The drawing under review shows one solid part. Ordinate dimensions are in mm from its lowest x, y, z. A direction names the side the tool comes from. Give positions to 0.01 mm unless a question says otherwise; leave off trailing zeros. Write each loop counter-clockwise with the first axis right and the second up, starting at its lowest first coordinate (ties: lowest second). Pieces come first, ordered by that corner, then holes. Notation, with made-up numbers: M 7,-17 L 12,-17 A22 cw 12,14 Z; hole C 52,-1 d6. An arc over 180 degrees is marked long. Write item = value, one per line. Start each with the question number.
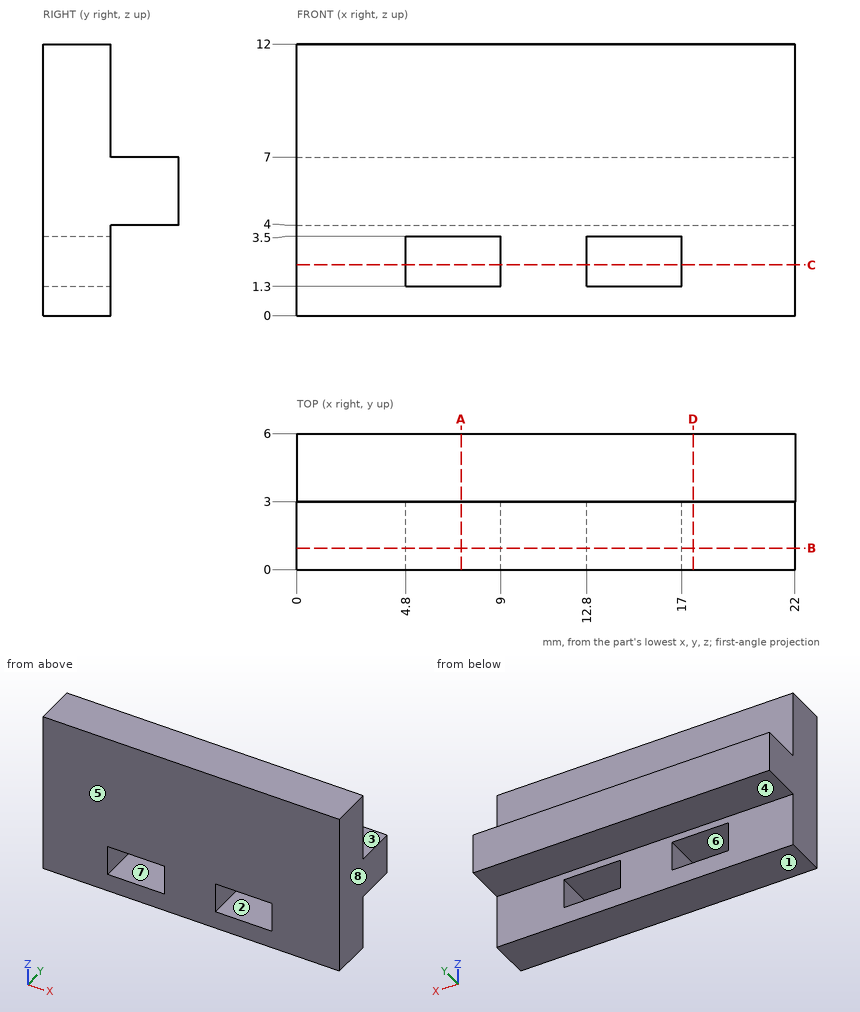
Item 1: To check wall thickness, follow probe 1 along X at (y, z) = (1.5, 3.25); probe 2 along Z at (x, y) = (15.5, 1.15); probe 3 along Z at (x, y) = (7.5, 4.45). State the ranges of each line that lie inside material, in increasing order. Write a range as [from, to].
Item 2: Clearance check with flat-ended pins moving along their axes: P1, Ø2.5, axis at x = 12, z = 10, coming from the +Y side; P2, Ø1.5, axis at x = 6.5, y = 4, coming from the +Z side. State where each tip first meets the part, or that it passes through.
Item 3: We need section C-C, the plane z = 2.25. Write out the cut boundary in (x, y).
Item 4: For the marked faces 1, 2, 3 and 4, list the 3-axis set-ups (+Z, -Z, +X, -X, +Y, -Y) from which the entire face can be reached by the end or side of a thin tool; tool diameter is ignored.
Item 5: We need section B-B, the plane y = 0.95. Write out the cut boundary in (x, z).
Item 6: The part is to be moulded in two halves that separate along X. For the marked faces 5, 6, 7 and 8, say which applies: released by +X, released by -X, zero draft, split by the parting line, or undercut.
Item 7: We need section D-D, the plane x = 17.5. Write out the cut boundary in (y, z).
Item 8: We need section A-A, the plane x = 7.25. Write out the cut boundary in (y, z).
Worked out:
q1.probe_1 = [0, 4.8], [9, 12.8], [17, 22]
q1.probe_2 = [0, 1.3], [3.5, 12]
q1.probe_3 = [4, 7]
q2.P1 = 3
q2.P2 = 7
q3.outline = M 0,0 L 4.8,0 L 4.8,3 L 0,3 Z; M 9,0 L 12.8,0 L 12.8,3 L 9,3 Z; M 17,0 L 22,0 L 22,3 L 17,3 Z
q4.face_1 = -Z, +X, -X, +Y, -Y
q4.face_2 = +Y, -Y
q4.face_3 = +Z, +X, -X, +Y
q4.face_4 = -Z, +X, -X, +Y
q5.outline = M 0,0 L 22,0 L 22,12 L 0,12 Z; hole M 4.8,1.3 L 9,1.3 L 9,3.5 L 4.8,3.5 Z; hole M 12.8,1.3 L 17,1.3 L 17,3.5 L 12.8,3.5 Z
q6.face_5 = zero draft
q6.face_6 = undercut
q6.face_7 = undercut
q6.face_8 = released by +X
q7.outline = M 0,0 L 3,0 L 3,4 L 6,4 L 6,7 L 3,7 L 3,12 L 0,12 Z
q8.outline = M 0,0 L 3,0 L 3,1.3 L 0,1.3 Z; M 0,3.5 L 3,3.5 L 3,4 L 6,4 L 6,7 L 3,7 L 3,12 L 0,12 Z
